The drawing under review shows one solid part. Ordinate dimensions are in mm from its lowest x, y, z. A direction names the side the tool comes from. Coordinates: 2 decimals unless noted, no trailing zeros. Write each loop counter-clockwise with the first axis right and the second up, starting at its lowest first coordinate (ties: lowest second). Pieces come first, ordered by that corner, then holes.
1) For the marked faces 1 and 2, list the 3-axis set-ups (+Z, -Z, +X, -X, +Y, -Y) from which the entire face can be reached by the end or side of a thin tool; tool diameter is ignored.
2) We need section C-C on y = 1.5. Write out the cut boundary in (x, z).
3) We need section A-A on y = 9.9. Write out the cut boundary in (x, z), then the cut area to 3 significant figures.
4) We need section D-D on z = 0.6. Write out the cut boundary in (x, y), then the cut area to 3 significant figures.
5) Mouldability with a two-part tool opening along Y and no side actions: class the marked faces 3, 4 and 5 as pulls with the +Y half, pulls with the -Y half, needs draft (parallel to the pull), parting line crosses it, or undercut.
6) Insertion check: P1, Ø2, axis at y = 14.5, z = 0.5, coming from the +X side; P2, Ø1.5, axis at y = 12.5, z = 4, coming from the -X side; P3, Ø3, axis at x = 3, z = 5, coming from the +Y side. Each pin has a flat end and moves straight along its axis. Give the tip position at first contact, or say it passes through.
7) To check wall thickness, follow line 1 along Y through (x, z) = (9.9, 2.95); line 2 along Y through (x, z) = (9.9, 1.5). State the ranges of each line that lie inside material, in increasing order.
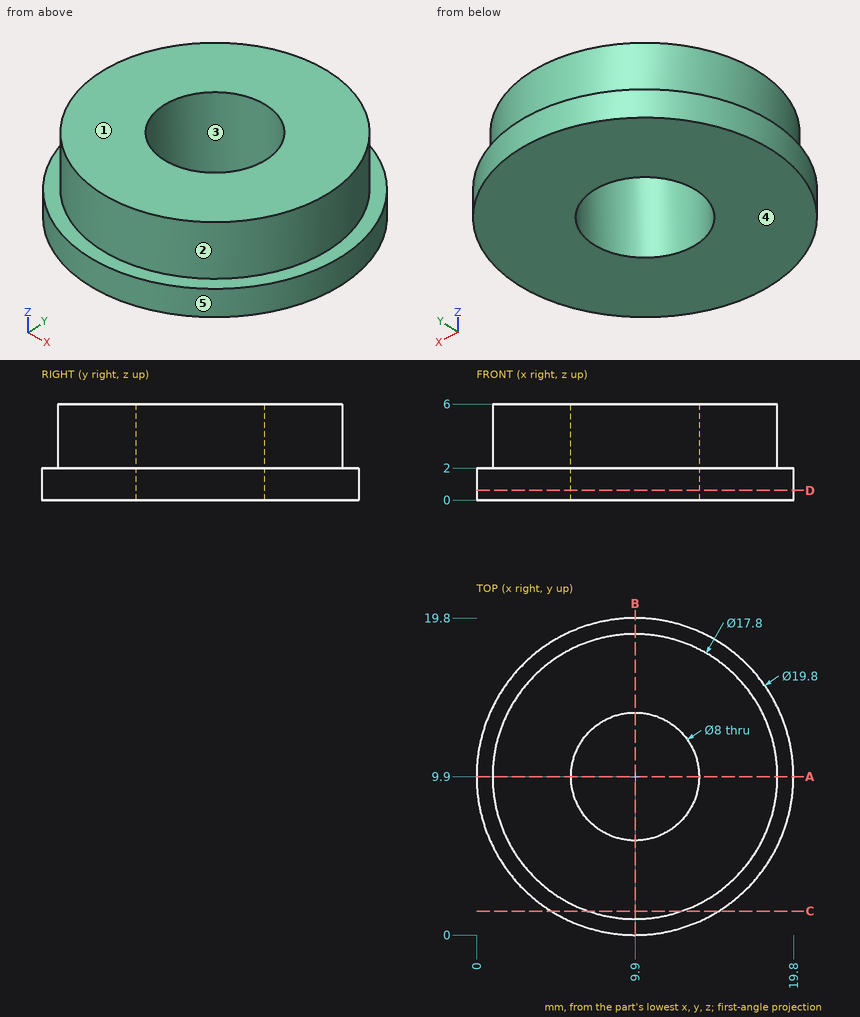
Result:
1. face 1: +Z, +X, -X, +Y, -Y
1. face 2: +Z
2. outline: (4.66, 0) - (15.14, 0) - (15.14, 2) - (12.84, 2) - (12.84, 6) - (6.96, 6) - (6.96, 2) - (4.66, 2) - close
3. outline: (0, 0) - (5.9, 0) - (5.9, 6) - (1, 6) - (1, 2) - (0, 2) - close; (13.9, 0) - (19.8, 0) - (19.8, 2) - (18.8, 2) - (18.8, 6) - (13.9, 6) - close
3. area: 62.8 mm2
4. outline: circle Ø19.8 at (9.9, 9.9); hole circle Ø8 at (9.9, 9.9)
4. area: 258 mm2
5. face 3: undercut
5. face 4: needs draft
5. face 5: parting line crosses it
6. P1: stops at x = 19.12
6. P2: stops at x = 1.19
6. P3: stops at y = 16.97
7. line 1: y = 1 to 5.9, 13.9 to 18.8
7. line 2: y = 0 to 5.9, 13.9 to 19.8
